```python
from build123d import *

# Parameters (mm, degrees)
SKETCH1_R           = 6
SKETCH1_R_2         = 1.75
BOSS_EXTRUDE1_DEPTH = 0.5
SKETCH2_R           = 6
SKETCH2_R_2         = 3.375
BOSS_EXTRUDE2_DEPTH = 1.5
FILLET1_R           = 0.25


with BuildPart() as part:
    # Sketch1 → Boss-Extrude1 (new body)
    with BuildSketch(Plane.XY):
        with Locations((-0.053524078, 0)):
            Circle(SKETCH1_R)
        Circle(SKETCH1_R_2, mode=Mode.SUBTRACT)
    extrude(amount=BOSS_EXTRUDE1_DEPTH)

    # Sketch2 → Boss-Extrude2 (add)
    with BuildSketch(Plane.XY.offset(0.5)):
        with Locations((-0.053524078, 0)):
            Circle(SKETCH2_R)
        Circle(SKETCH2_R_2, mode=Mode.SUBTRACT)
    extrude(amount=BOSS_EXTRUDE2_DEPTH)

    # Fillet1
    fillet1_edges = [part.edges().sort_by_distance(p)[0] for p in [
        (-6.053524078, 0, 2),
        (-6.053524078, 0, 0),
    ]]
    fillet(fillet1_edges, radius=FILLET1_R)


solid = part.part
```
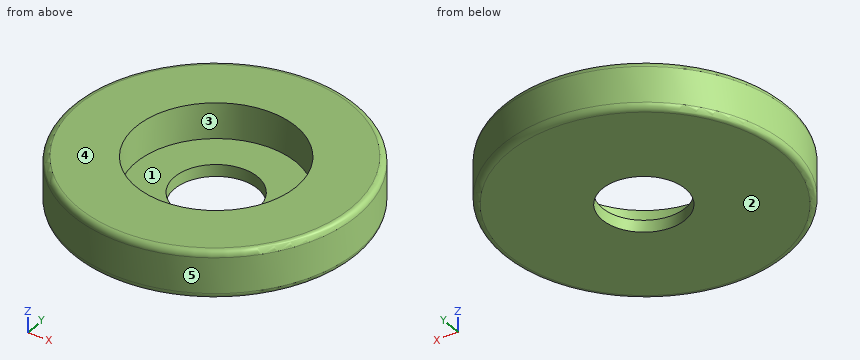
Part model, mm, in its own coordinate system. Face numbers are marked on the shaded views. A direction names the side the tool comes from. Round coordinates to 2 decimals unless told otherwise and drop trailing zeros. Loops run counter-clockwise (first coordinate to the right, second up) from the corner with the lowest first, then second, coordinate; pieces in that order, holes last.
1. Slice it at B-B (z = 1.4). Give the cut face in (x, y) (3 decimals).
Solutions:
outline: circle Ø12 at (-0.054, 0); hole circle Ø6.75 at (0, 0)
2. 3-axis set-ups, long thin cutter, end or side, ignore diameter. For the marked faces 1 and 2: which of +Z, -Z, +X, -X, +Y, -Y reach the whole face in a straight line?
Solutions:
face 1: +Z
face 2: -Z, +X, -X, +Y, -Y
3. Flat gauge pins, fed straight in: pin 1 (5.5 mm diameter, centred on x = 0, y = 0, fed in from +Z); pin 2 (1 mm diameter, centred on y = -1.5, z = 1.5, fed in from -X). Where does each tip first touch, or does it go through?
Solutions:
pin 1: stops at z = 0.5
pin 2: stops at x = -5.97
4. Drill centre lines: line 1 along Z through (x, y) = (1.5, -2); line 2 along X through (y, z) = (2, 1.15); line 3 along Y through (x, z) = (0, 1.25) (3 decimals). Where is each one in solid material? Low to high.
Solutions:
line 1: z = 0 to 0.5
line 2: x = -5.71 to -2.72, 2.72 to 5.6
line 3: y = -6 to -3.375, 3.375 to 6
5. Slice it at A-A (y = 0). Give the cut face in (x, z) (3 decimals), and give its area (3 significant figures).
Solutions:
outline: (-6.054, 0.25) arc R0.25 ccw to (-5.804, 0) - (-1.75, 0) - (-1.75, 0.5) - (-3.375, 0.5) - (-3.375, 2) - (-5.804, 2) arc R0.25 ccw to (-6.054, 1.75) - close; (1.75, 0) - (5.696, 0) arc R0.25 ccw to (5.946, 0.25) - (5.946, 1.75) arc R0.25 ccw to (5.696, 2) - (3.375, 2) - (3.375, 0.5) - (1.75, 0.5) - close
area: 12.1 mm2
6. Two-plate mould, pull along Y, no slides. Class the marked faces 3, 4 and 5: pulls with the +Y half, pulls with the -Y half, needs draft (parallel to the pull), parting line crosses it, or undercut.
Solutions:
face 3: undercut
face 4: needs draft
face 5: parting line crosses it
